from build123d import *

# Parameters (mm, degrees)
BASE_EXTRUSION_DEPTH    = 12
ESQUISSE3_R             = 10
ENL_V_MAT_EXTRU_1_DEPTH = 26.865034313


with BuildPart() as part:
    # Esquisse1 → Base-Extrusion (new body)
    with BuildSketch(Plane.XY):
        Polygon((15, -8.660254038), (15, 8.660254038), (0, 17.320508076), (-15, 8.660254038), (-15, -8.660254038), (0, -17.320508076), align=None)
    extrude(amount=-BASE_EXTRUSION_DEPTH)

    # Esquisse2 → Enlèvement de matière-Révolution1 (revolve, cut)
    with BuildSketch(Plane(origin=(0, 0, 0), x_dir=(1, 0, 0), z_dir=(0, 1, 0))):
        Polygon((-15, 0), (-26.392304845, 0), (-26.392304845, 12), (-15, 12), (-25.392304845, 6), align=None)
    revolve(axis=Axis((0, 0, -12), (0, 0, 1)), mode=Mode.SUBTRACT)

    # Esquisse3 → Enlèv. mat.-Extru.1 (cut, through all)
    with BuildSketch(Plane.XY):
        Circle(ESQUISSE3_R)
    extrude(amount=-ENL_V_MAT_EXTRU_1_DEPTH, mode=Mode.SUBTRACT)


solid = part.part
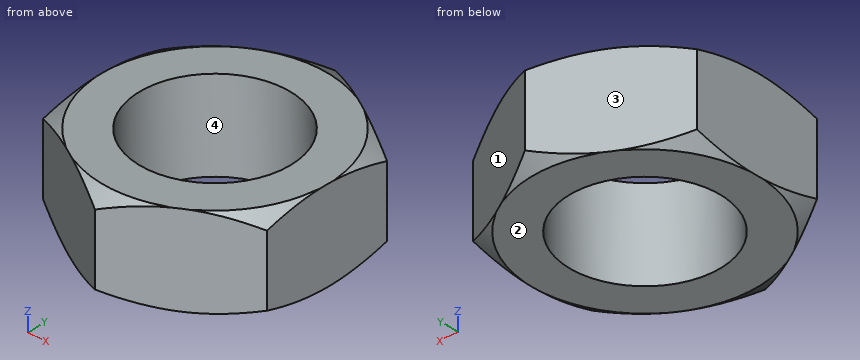
Source: CAD feature listing. Evaluate the final solid. Frame: model axes, mm. Face numbers are marked on the shaded views. Coordinates: 2 decimals unless noted, no trailing zeros. Loops run counter-clockwise (first coordinate to the right, second up) from the corner with the lowest first, then second, coordinate; pieces in that order, holes last. Notation, with made-up numbers: (31, -24) - (79, -24) arc R17 cw to (79, 1) - close; hole circle Ø11 at (89.25, 2.25). An arc over 180 degrees is marked (long way). Return JSON: item names as keys, results as strings.
Q1. Contact query for flat-ended pins moving along their axis: P1, Ø3, axis at x = -5.5, z = -8.5, coming from the -Y side; P2, Ø3, axis at y = 13.5, z = -8, coming from the +X side; P3, Ø2, axis at x = 9, z = -8.5, coming from the +Y side. Output: stop coordinate, or through.
Results:
{"P1": "y = -15.01", "P2": "x = 9.22", "P3": "y = 12.7"}
Q2. Mould query, pull axis X, two halves, no side actions, for the marked faces 1, 2, 3 and 4. Classes: released by +X, released by -X, zero draft, split by the parting line, or undercut.
Results:
{"face 1": "released by +X", "face 2": "zero draft", "face 3": "released by -X", "face 4": "undercut"}
Q3. Material intervals for line 1 along Y through (x, z) = (0, -6); line 2 along Y through (x, z) = (0.5, -2); line 3 along X through (y, z) = (-6, -4.75), sorted ascending.
Results:
{"line 1": "-17.32 to -10, 10 to 17.32", "line 2": "-17.03 to -9.99, 9.99 to 17.03", "line 3": "-15 to -8, 8 to 15"}
Q4. Section A-A, the plane z = -9. Return loops of the section in (x, y).
Results:
{"outline": "(-15, -8.66) - (0, -17.32) - (15, -8.66) - (15, 8.66) - (0, 17.32) - (-15, 8.66) - close; hole circle Ø20 at (0, 0)"}
